from build123d import *

# Parameters (mm, degrees)
F1_DEPTH     = 31.75
F2_T1_DEPTH  = 42.6160723951
F2_T3_DEPTH  = 41.3681408406
F2_T8_ANGLE  = 42.4045514756
F2_T13_ANGLE = 42.4045514756
F2_T18_ANGLE = 105.7775701063
F2_T23_ANGLE = 105.7775701063
F2_T28_DEPTH = 21.5661635602
F2_T33_DEPTH = 21.5661635602
F3_R         = 3.81


# Not quite as in the source:
# - a fillet or chamfer that OpenCascade refuses, or shapes differently, is made with other operations: its cross-section is extruded or revolved along the edge and cut away or added


with BuildPart() as f1:
    # F0 (on Front) → F1 (new body)
    with BuildSketch(Plane.XZ):
        with BuildLine():
            Line((-34.918975085, 0), (0, 0))
            Line((0, 0), (41.5991283953, 0))
            Line((41.5991283953, 0), (41.5991283953, 7.7429031953))
            ThreePointArc((41.5991283953, 7.7429031953), (24.4471014125, 13.2848832085), (9.4129433855, 23.2287086546))
            Line((9.4129433855, 23.2287086546), (21.2550275028, 23.2287086546))
            Line((21.2550275028, 23.2287086546), (21.2550275028, 31.730722636))
            Line((21.2550275028, 31.730722636), (8.8056568056, 31.730722636))
            Line((8.8056568056, 31.730722636), (37.6517660916, 35.6780849397))
            Line((37.6517660916, 35.6780849397), (37.6517660916, 46.912882477))
            Line((37.6517660916, 46.912882477), (-25.8096773177, 46.912882477))
            Line((-25.8096773177, 46.912882477), (-32.4898287654, 40.8400185406))
            Line((-32.4898287654, 40.8400185406), (-27.3100329334, 35.1422421722))
            Line((-27.3100329334, 35.1422421722), (-20.3440990299, 32.3380082846))
            Line((-20.3440990299, 32.3380082846), (-29.4533986598, 32.3380082846))
            Line((-29.4533986598, 32.3380082846), (-29.4533986598, 25.0505693257))
            Line((-29.4533986598, 25.0505693257), (-20.3440990299, 25.0505693257))
            ThreePointArc((-20.3440990299, 25.0505693257), (-24.9642185282, 14.1505733942), (-34.918975085, 7.7429031953))
            Line((-34.918975085, 7.7429031953), (-34.918975085, 0))
        make_face()
    extrude(amount=F1_DEPTH)

    # F2: chamfer of 2.54 on 8 edges, made by hand

    # F2_s2 → F2_t1 (cut)
    with BuildSketch(Plane.XZ.offset(-5.4330361975)):
        with BuildLine():
            Line((39.5823851634, 8.1350460371), (41.5991283953, 5.6495275088))
            Line((41.5991283953, 5.6495275088), (41.5991283953, 7.7429031953))
            ThreePointArc((41.5991283953, 7.7429031953), (40.55098868, 7.9386371476), (39.5823851634, 8.1350460371))
        make_face()
    extrude(amount=F2_T1_DEPTH, mode=Mode.SUBTRACT)

    # F2_s4 → F2_t3 (cut)
    with BuildSketch(Plane.XZ.offset(-4.8090704203)):
        with BuildLine():
            Line((-34.918975085, 5.9036651076), (-33.2718375789, 8.2815626174))
            ThreePointArc((-33.2718375789, 8.2815626174), (-34.0510462722, 8.0071201362), (-34.918975085, 7.7429031953))
            Line((-34.918975085, 7.7429031953), (-34.918975085, 5.9036651076))
        make_face()
    extrude(amount=F2_T3_DEPTH, mode=Mode.SUBTRACT)


with BuildPart() as f2_tool6:
    # F2_s7 → F2_t8 (revolve)
    with BuildSketch(Plane(origin=(47.2414051796, 0, -3.7108637316), x_dir=(0, 1, 0), z_dir=(0.9969290674, 0, -0.078309862))):
        Polygon((-31.75, 8.1162253666), (-29.21, 10.6562253666), (-31.75, 10.6562253666), align=None)
    revolve(axis=Axis((53.2845253443, -31.75, 73.221491886), (0, 1, 0)), revolution_arc=F2_T8_ANGLE)

    split(bisect_by=Plane.XY.offset(23.2287086546), keep=Keep.BOTTOM)


with BuildPart() as f1_1:
    add(f1.part)

    # F2_t5: cut F2_tool6
    add(f2_tool6.part, mode=Mode.SUBTRACT)


with BuildPart() as f2_tool11:
    # F2_s12 → F2_t13 (revolve)
    with BuildSketch(Plane(origin=(47.2414051796, 0, -3.7108637316), x_dir=(0, 1, 0), z_dir=(0.9969290674, 0, -0.078309862))):
        Polygon((-2.54, 10.6562253666), (0, 8.1162253666), (0, 10.6562253666), align=None)
    revolve(axis=Axis((53.2845253443, 0, 73.221491886), (0, 1, 0)), revolution_arc=F2_T13_ANGLE)

    split(bisect_by=Plane.XY.offset(23.2287086546), keep=Keep.BOTTOM)


with BuildPart() as f1_2:
    add(f1_1.part)

    # F2_t10: cut F2_tool11
    add(f2_tool11.part, mode=Mode.SUBTRACT)


with BuildPart() as f2_tool16:
    # F2_s17 → F2_t18 (revolve)
    with BuildSketch(Plane(origin=(-7.8247411196, 0, 34.4744832645), x_dir=(0, 1, 0), z_dir=(-0.2213421957, 0, 0.975196202))):
        Polygon((-31.75, 10.7019792675), (-29.21, 13.2419792675), (-31.75, 13.2419792675), align=None)
    revolve(axis=Axis((-40.3361011805, -31.75, 27.0953160709), (0, 1, 0)), revolution_arc=F2_T18_ANGLE)

    split(bisect_by=Plane.XY.offset(25.0505693257), keep=Keep.BOTTOM)


with BuildPart() as f1_3:
    add(f1_2.part)

    # F2_t15: cut F2_tool16
    add(f2_tool16.part, mode=Mode.SUBTRACT)


with BuildPart() as f2_tool21:
    # F2_s22 → F2_t23 (revolve)
    with BuildSketch(Plane(origin=(-7.8247411196, 0, 34.4744832645), x_dir=(0, 1, 0), z_dir=(-0.2213421957, 0, 0.975196202))):
        Polygon((-2.54, 13.2419792675), (0, 10.7019792675), (0, 13.2419792675), align=None)
    revolve(axis=Axis((-40.3361011805, 0, 27.0953160709), (0, 1, 0)), revolution_arc=F2_T23_ANGLE)

    split(bisect_by=Plane.XY.offset(25.0505693257), keep=Keep.BOTTOM)


with BuildPart() as f1_4:
    add(f1_3.part)

    # F2_t20: cut F2_tool21
    add(f2_tool21.part, mode=Mode.SUBTRACT)


with BuildPart() as f2_tool26:
    # F2_s27 → F2_t28 (new body)
    with BuildSketch(Plane.XY.offset(16.6966338652)):
        Polygon((18.7150275028, 0), (21.2550275028, -2.54), (21.2550275028, 0), align=None)
    extrude(amount=F2_T28_DEPTH)

    split(bisect_by=Plane(origin=(-4.1004226977, 0, 29.9646275548), x_dir=(0, 1, 0), z_dir=(0.1355785861, 0, -0.9907665956)), keep=Keep.TOP)


with BuildPart() as f1_5:
    add(f1_4.part)

    # F2_t25: cut F2_tool26
    add(f2_tool26.part, mode=Mode.SUBTRACT)


with BuildPart() as f2_tool31:
    # F2_s32 → F2_t33 (new body)
    with BuildSketch(Plane.XY.offset(16.6966338652)):
        Polygon((18.7150275028, -31.75), (21.2550275028, -29.21), (21.2550275028, -31.75), align=None)
    extrude(amount=F2_T33_DEPTH)

    split(bisect_by=Plane(origin=(-4.1004226977, 0, 29.9646275548), x_dir=(0, 1, 0), z_dir=(0.1355785861, 0, -0.9907665956)), keep=Keep.TOP)


with BuildPart() as f1_6:
    add(f1_5.part)

    # F2_t30: cut F2_tool31
    add(f2_tool31.part, mode=Mode.SUBTRACT)

    # F3
    f3_edges = [f1_6.edges().sort_by_distance(p)[0] for p in [
        (-29.453399, -31.75, 28.694289),
        (-29.453399, 0, 28.694289),
        (37.651766, -15.875, 46.912882),
    ]]
    fillet(f3_edges, radius=F3_R)


solid = f1_6.part
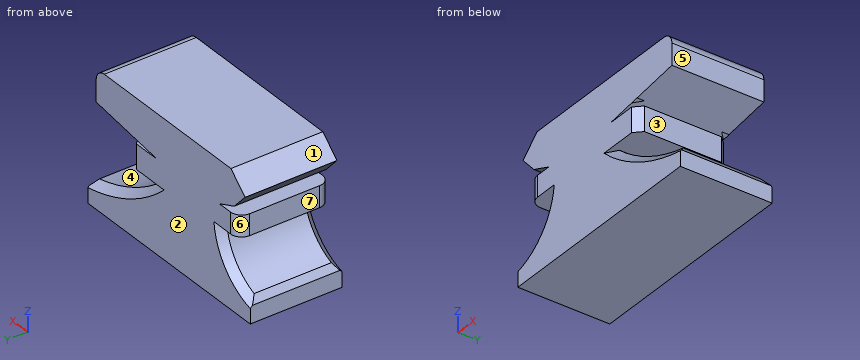
Can you work these out from the model? Positions are in its coordinate system, mm. Face numbers are marked on the shaded views. A direction names the side the tool comes from. Give positions to 0.01 mm unless a question says otherwise; leave off trailing zeros. Order: outer loops, then holes, each group sorted by start corner. A loop starts at its lowest first (then second) coordinate and runs counter-clockwise, first axis right, second up. Notation, with made-up numbers: (-22.75, -36.75) - (-12.75, -36.75) arc R34 ccw to (-12.75, -5.75) - close; hole circle Ø6 at (40, 13). An arc over 180 degrees is marked (long way). Write each question's results on one line, items separated by ' | '.
1) Please list where these lines run through material, in increasing order: line 1 along Z through (x, y) = (18, -19); line 2 along Z through (x, y) = (-27, -25); line 3 along Z through (x, y) = (26.5, -5). Write a range as [from, to].
Final values:
line 1: z = [0, 16.84], [23.23, 31.73], [32.99, 46.91] | line 2: z = [0, 12.06], [25.05, 32.34], [35.02, 45.83] | line 3: z = [0, 12.34], [34.15, 46.91]
2) If we mould it in two halves opening along Z, with no side actions, what happens to the marked faces 1, 2, 3 and 4? For each: pulls with the +Z half, pulls with the -Z half, needs draft (parallel to the pull), parting line crosses it, or undercut.
Final values:
face 1: pulls with the +Z half | face 2: needs draft | face 3: undercut | face 4: undercut
3) Suppose I cut it at B-B, the plane y = -25. Write out the boundary of the cut face in (x, z).
Final values:
outline: (-34.92, 0) - (41.6, 0) - (41.6, 5.65) - (39.58, 8.14) arc R66.51 cw to (9.41, 23.23) - (21.26, 23.23) - (21.26, 31.73) - (8.81, 31.73) - (37.65, 35.68) - (37.65, 43.1) arc R3.81 ccw to (33.84, 46.91) - (-25.81, 46.91) - (-32.49, 40.84) - (-27.31, 35.14) - (-20.34, 32.34) - (-29.45, 32.34) - (-29.45, 25.05) - (-20.34, 25.05) arc R20.1 cw to (-33.27, 8.28) - (-34.92, 5.9) - close
4) I'm going to push flat-ended pins straight in: pin 1 Ø7 at (y, z) = (-14, 27.5) entering from +X (3 decimals); pin 2 Ø2 at (y, z) = (-12.5, 28) entering from -X; pin 3 Ø8 at (y, z) = (-3.5, 34.5) entering from +X. Where does each tip first touch, or does it pass through?
Final values:
pin 1: stops at x = 21.255 | pin 2: stops at x = -29.45 | pin 3: stops at x = 37.65
5) Suppose I cut it at A-A, the plane z = 28. Write out the boundary of the cut face in (x, y).
Final values:
outline: (-29.45, -27.94) arc R3.81 ccw to (-25.64, -31.75) - (18.72, -31.75) - (21.26, -29.21) - (21.26, -2.54) - (18.72, 0) - (-25.64, 0) arc R3.81 ccw to (-29.45, -3.81) - close
6) On a 3-axis mill with a long thin cutter (end or side, diameter ignored), from which of +Z, -Z, +X, -X, +Y, -Y can I reach the whole of each face in a straight line? I mean the marked faces 5, 6 and 7. Say none if no direction works.
Final values:
face 5: +Z, +X, +Y, -Y | face 6: -X, +Y | face 7: -X, +Y, -Y
